from build123d import *

# Parameters (mm, degrees)
F1_DEPTH = 100
F2_R     = 6
F3_R     = 12


with BuildPart() as f1:
    # F0 (on Top) → F1 (new body)
    with BuildSketch(Plane.XY):
        Polygon((0, 6), (0, 0), (32.5, 0), (32.5, 30), (26.5, 30), (26.5, 6), align=None)
        Polygon((-32.5, 0), (0, 0), (0, 6), (-26.5, 6), (-26.5, 30), (-32.5, 30), align=None)
    extrude(amount=F1_DEPTH)

    # F2
    f2_edges = [f1.edges().sort_by_distance(p)[0] for p in [
        (26.5, 6, 50),
        (-26.5, 6, 50),
    ]]
    fillet(f2_edges, radius=F2_R)

    # F3
    f3_edges = [f1.edges().sort_by_distance(p)[0] for p in [
        (32.5, 0, 50),
        (-32.5, 0, 50),
    ]]
    fillet(f3_edges, radius=F3_R)


solid = f1.part
Can you work these out from the model? Positions are in its coordinate system, mm. A direction names the side the tool comes from. Coordinates: 2 decimals unless noted, no trailing zeros. Write each loop counter-clockwise with the first axis right and the second up, starting at its lowest first coordinate (ties: lowest second). Pieces come first, ordered by that corner, then holes. Notation, with made-up numbers: (47, 27.5) -> (99, 27.5) arc R20 ccw to (99, 64.5) -> close; hole circle Ø10 at (58.5, -6.5). An arc over 180 degrees is marked (long way). Answer as CSV lines item,"result".
1) If I drill on line 1 (X direction, y = 19.5, z = 83.5); line 2 (Y direction, x = 12, z = 7.5); line 3 (X direction, y = 10.75, z = 47.5), over which ranges is the centre line in solid material (lowest first)? Write a range as from..to.
Check result:
line 1,"-32.5..-26.5, 26.5..32.5"
line 2,"0..6"
line 3,"-32.43..-26.37, 26.37..32.43"
2) On a 3-axis mill with a long thin cutter (end or side, diameter ignored), from which of +Z, -Z, +X, -X, +Y, -Y can I reach the whole of each face in a straight line? I mean faces 5 (the flat face through (0, 5, 100)), 6 (the flat face through (0, 6, 49)). Say none if no direction works.
Check result:
face 5,"+Z, +X, -X, +Y, -Y"
face 6,"+Z, -Z, +Y"
3) Will these pins go through, and if not, where does the flat tip stop? P1, Ø3, axis at y = 5, z = 42.5, coming from the +X side; P2, Ø20.5, axis at x = -5, z = 52.5, coming from the +Y side.
Check result:
P1,"x = 31.17"
P2,"y = 6"
4) If we section it at D-D on y = 9: Please give me the cut outline in (x, z), then the cut area to 3 significant figures.
Check result:
outline,"(-32.12, 0) -> (-25.7, 0) -> (-25.7, 100) -> (-32.12, 100) -> close; (25.7, 0) -> (32.12, 0) -> (32.12, 100) -> (25.7, 100) -> close"
area,"1,280 mm²"
5) If we section it at C-C on x = 17: Please give me the cut outline in (y, z).
Check result:
outline,"(0, 0) -> (6, 0) -> (6, 100) -> (0, 100) -> close"
6) If we section it at B-B on z = 12.5: Please give me the cut outline in (x, y), then the cut area to 3 significant figures.
Check result:
outline,"(-32.5, 12) arc R12 ccw to (-20.5, 0) -> (20.5, 0) arc R12 ccw to (32.5, 12) -> (32.5, 30) -> (26.5, 30) -> (26.5, 12) arc R6 cw to (20.5, 6) -> (-20.5, 6) arc R6 cw to (-26.5, 12) -> (-26.5, 30) -> (-32.5, 30) -> close"
area,"632 mm²"
7) If we section it at A-A on y = 20.75: Please give me the cut outline in (x, z), then the cut area to 3 significant figures.
Check result:
outline,"(-32.5, 0) -> (-26.5, 0) -> (-26.5, 100) -> (-32.5, 100) -> close; (26.5, 0) -> (32.5, 0) -> (32.5, 100) -> (26.5, 100) -> close"
area,"1,200 mm²"
8) If we mould it in two halves opening along X, with no side actions, what happens to faces 1 (the cylindrical face through (29.08, 3.61, 50.7)), 2 (the flat face through (-32.5, 21, 49)), 3 (the cylindrical face through (24.789, 7.804, 50.7)), 4 (the flat face through (-29, 30, 49))? For each: +X half, -X half, draft (parallel to the pull), parting line (faces both ways), or undercut.
Check result:
face 1,"+X half"
face 2,"-X half"
face 3,"undercut"
face 4,"draft"
